Geometry: final body of the model. Coordinates: model frame, mm. Face numbers are marked on the shaded views. A direction names the side the tool comes from. Coordinates: 2 decimals unless noted, no trailing zeros. Order: outer loops, then holes, each group sorted by start corner. A loop starts at its lowest first (then second) coordinate and runs counter-clockwise, first axis right, second up. Notation, with made-up numbers: M -17,-39.5 L 18,-39.5 A20 cw 18,-25.5 Z; hole C 89,73.25 d3. An arc over 180 degrees is marked long. Use CSV: the item, a comma, the result in double quotes. Start each with the question number.
Q1. Section query D-D, the plane z = 63.5. Output: boundary loops of the cut face in (x, y), and give its area (3 significant figures).
Q2. First-contact query: P1, Ø5, axis at x = -22, z = -16, coming from the +Y side; P2, Ø3, axis at y = 90.65, z = -0.1, coming from the +X side. Flat tips, straight axial feed; report the tip coordinate or a pass-through.
Q3. Section query A-A, the plane y = 73.5. Output: boundary loops of the cut face in (x, z), and give its area (3 significant figures).
Q4. Ray query, probe 1 along X at (y, z) = (11.5, 0); probe 2 along Z at (x, y) = (74.25, 90.65); probe 3 along Y at (x, z) = (-73.5, -0.1). Return the intervals inside material, ascending.
Q5. Mould query, pull axis Z, two halves, no side actions, for the marked faces 3, 4, 5 and 6. Classes: +Z half, -Z half, draft (parallel to the pull), parting line (faces both ways), or undercut.
Q6. Section query B-B, the plane x = 0. Output: boundary loops of the cut face in (y, z), and give its area (3 significant figures).
Q7. Section query C-C, the plane z = -7.5. Output: boundary loops of the cut face in (x, y), and give its area (3 significant figures).
Q8. Access query for the marked faces 1 and 2. Directions: +Z, -Z, +X, -X, +Y, -Y. A direction counts if a zero-diameter tool reaches every point of the face in a straight line with its end or side. Return the directions, or none.
from build123d import *

# Parameters (mm, degrees)
SKETCH_1_W          = 150
SKETCH_1_H          = 150
EXTRUDE_1_DEPTH     = 3
SKETCH_2_W          = 150
SKETCH_2_H          = 150
SKETCH_2_W_2        = 144
SKETCH_2_H_2        = 144
EXTRUDE_2_DEPTH     = 107.65
SKETCH_3_R          = 27.5
CUT_EXTRUDE_1_DEPTH = 91
SKETCH_4_R          = 4
CUT_EXTRUDE_2_DEPTH = 201.9189451
SKETCH_8_R          = 35
SKETCH_8_R_2        = 31.25
EXTRUDE_4_DEPTH     = 14
SKETCH_9_R          = 1.65
CUT_EXTRUDE_3_DEPTH = 201.9189451


with BuildPart() as part:
    # 草图1 → 凸台-拉伸1 (new body)
    with BuildSketch(Plane(origin=(0, 0, 0), x_dir=(1, 0, 0), z_dir=(0, 1, 0))):
        Rectangle(SKETCH_1_W, SKETCH_1_H)
    extrude(amount=EXTRUDE_1_DEPTH)

    # 草图2 → 凸台-拉伸2 (add)
    with BuildSketch(Plane(origin=(0, 3, 0), x_dir=(1, 0, 0), z_dir=(0, 1, 0))):
        Rectangle(SKETCH_2_W, SKETCH_2_H)
        Rectangle(SKETCH_2_W_2, SKETCH_2_H_2, mode=Mode.SUBTRACT)
    extrude(amount=EXTRUDE_2_DEPTH)

    # 草图3 → 切除-拉伸1 (cut)
    with BuildSketch(Plane.XZ):
        with Locations(Location((0, 0, 0), (0, 0, 270))):
            Circle(SKETCH_3_R)
    extrude(amount=-CUT_EXTRUDE_1_DEPTH, mode=Mode.SUBTRACT)

    # 草图4 → 切除-拉伸2 (cut, through all)
    with BuildSketch(Plane.ZY.offset(75)):
        with Locations((-20.1, 110.65)):
            Circle(SKETCH_4_R)
    extrude(amount=-CUT_EXTRUDE_2_DEPTH, mode=Mode.SUBTRACT)

    # 草图8 → 凸台-拉伸4 (add)
    with BuildSketch(Plane(origin=(0, 3, 0), x_dir=(1, 0, 0), z_dir=(0, 1, 0))):
        with Locations(Location((0, 0, 0), (0, 0, 270))):
            Circle(SKETCH_8_R)
        with Locations(Location((0, 0, 0), (0, 0, 270))):
            Circle(SKETCH_8_R_2, mode=Mode.SUBTRACT)
    extrude(amount=EXTRUDE_4_DEPTH)

    # 草图9 → 切除-拉伸3 (cut, through all)
    with BuildSketch(Plane.ZY.offset(75)):
        with Locations((-40.1, 90.65)):
            Circle(SKETCH_9_R)
        with Locations((-0.1, 90.65)):
            Circle(SKETCH_9_R)
    extrude(amount=-CUT_EXTRUDE_3_DEPTH, mode=Mode.SUBTRACT)


solid = part.part
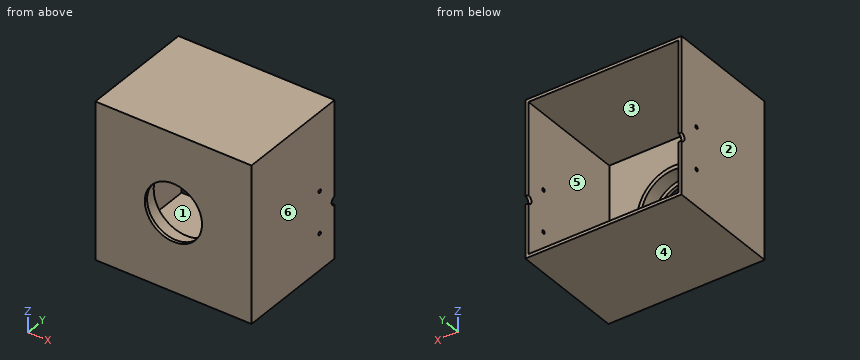
Responses:
1,outline,"M -75,0 L 75,0 L 75,110.65 L 72,110.65 L 72,3 L -72,3 L -72,110.65 L -75,110.65 Z"
1,area,"1,100 mm²"
2,P1,"stops at y = 3"
2,P2,"passes through"
3,outline,"M -75,-75 L 75,-75 L 75,75 L -75,75 Z; hole M -72,-72 L 72,-72 L 72,72 L -72,72 Z"
3,area,"1,760 mm²"
4,probe 1,"x = -75 to -72, -35 to -31.25, 31.25 to 35, 72 to 75"
4,probe 2,"z = -75 to -41.75, -38.45 to -1.75, 1.55 to 75"
4,probe 3,"y = 0 to 89, 92.3 to 110.65"
5,face 3,"undercut"
5,face 4,"-Z half"
5,face 5,"undercut"
5,face 6,"draft"
6,outline,"M 0,-75 L 110.65,-75 L 110.65,-72 L 3,-72 L 3,-35 L 17,-35 L 17,-31.25 L 3,-31.25 L 3,-27.5 L 0,-27.5 Z; M 0,27.5 L 3,27.5 L 3,31.25 L 17,31.25 L 17,35 L 3,35 L 3,72 L 110.65,72 L 110.65,75 L 0,75 Z"
6,area,"1,040 mm²"
7,outline,"M -75,0 L -26.46,0 L -26.46,3 L -30.34,3 L -30.34,17 L -34.19,17 L -34.19,3 L -72,3 L -72,110.65 L -75,110.65 Z; M 26.46,0 L 75,0 L 75,110.65 L 72,110.65 L 72,3 L 34.19,3 L 34.19,17 L 30.34,17 L 30.34,3 L 26.46,3 Z"
7,area,"1,040 mm²"
8,face 1,"+Y"
8,face 2,"+Z, -Z, -X, +Y, -Y"
